Job drawing, mm, ordinate dimensions from the low corner. One solid piece. Round coordinates to 2 decimals unless told otherwise and drop trailing zeros. Order: outer loops, then holes, each group sorted by start corner. A loop starts at its lowest first (then second) coordinate and runs counter-clockwise, first axis right, second up. Notation, with made-up numbers: (-33.75, 82) -> (10.25, 82) arc R13 ccw to (10.25, 91) -> close; hole circle Ø6 at (14, 86). An arc over 180 degrees is marked (long way). Write item = value, one per line.
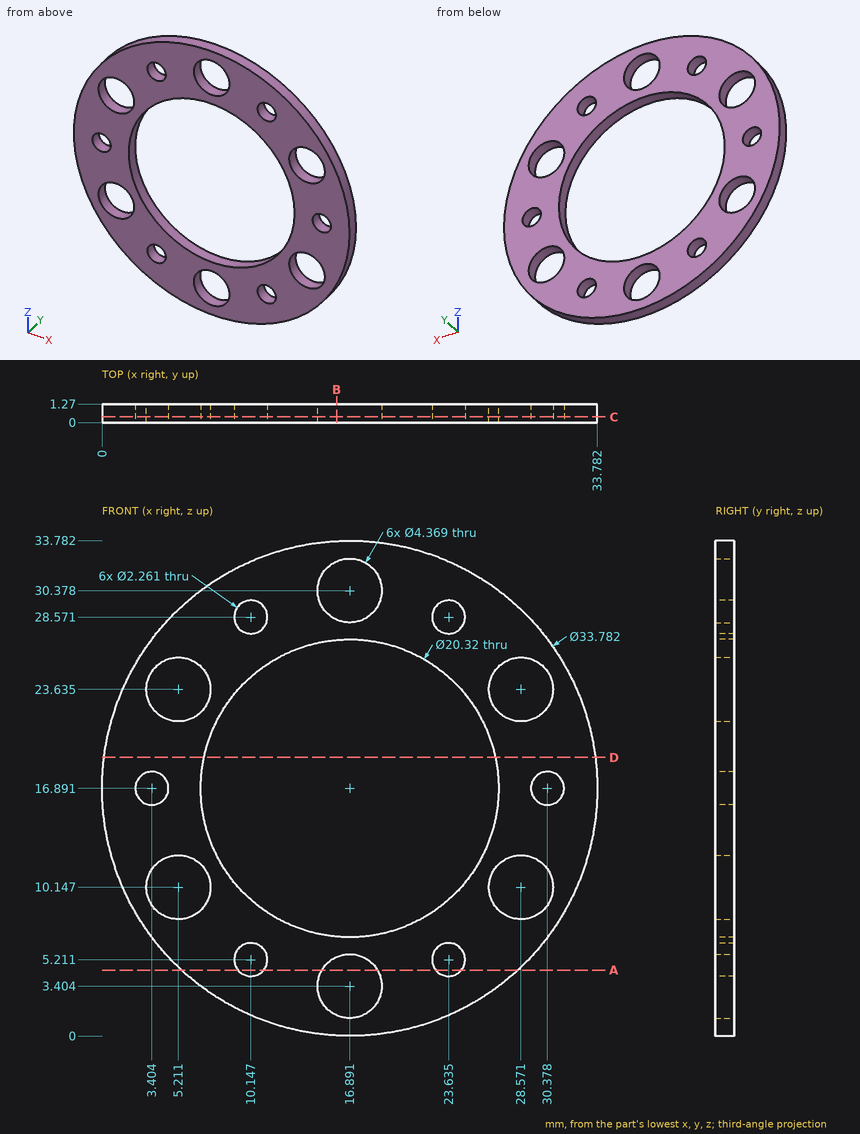
Q1. Cut at D-D, the plane z = 19. List the corners of the cut face in (x, y).
Check values:
outline = (0.13, 0) -> (6.95, 0) -> (6.95, 1.27) -> (0.13, 1.27) -> close; (26.83, 0) -> (33.65, 0) -> (33.65, 1.27) -> (26.83, 1.27) -> close
Q2. Cut at B-B, the plane x = 16. List the corners of the cut face in (y, z).
Check values:
outline = (0, 0.02) -> (1.27, 0.02) -> (1.27, 1.41) -> (0, 1.41) -> close; (0, 5.4) -> (1.27, 5.4) -> (1.27, 6.77) -> (0, 6.77) -> close; (0, 27.01) -> (1.27, 27.01) -> (1.27, 28.38) -> (0, 28.38) -> close; (0, 32.37) -> (1.27, 32.37) -> (1.27, 33.76) -> (0, 33.76) -> close
Q3. Probe probe 1 along X at (y, z) = (0.45, 10.5) (1 decimal); probe 2 along Z at (x, y) = (5, 1.2) (1 decimal); probe 3 along X at (y, z) = (0.9, 6) (1 decimal). List the from-to ranges inside material, lowest first.
Check values:
probe_1 = 1.3 to 3.1, 7.4 to 9, 24.8 to 26.4, 30.7 to 32.5
probe_2 = 4.9 to 8, 12.3 to 21.5, 25.8 to 28.9
probe_3 = 4 to 9.3, 11 to 22.8, 24.4 to 29.8
Q4. Flat gauge pin, fed straight in: pin 1 (2.5 mm diameter, centred on x = 30.38, z = 16.89, fed in from -Y). Where does the tip first touch, or does it go through?
Check values:
pin_1 = 0
Q5. Cut at C-C, the plane y = 0.4. Give the number of separate pieces and of enclosed holes in the cut face, and give its area (3 significant figures).
Check values:
separate_pieces = 1
enclosed_holes = 13
area = 458 mm²
Q6. Cut at A-A, the plane z = 4.5. List the corners of the cut face in (x, y) (1 decimal), and give its area (3 significant figures).
Check values:
outline = (5.4, 0) -> (9.3, 0) -> (9.3, 1.3) -> (5.4, 1.3) -> close; (11, 0) -> (15, 0) -> (15, 1.3) -> (11, 1.3) -> close; (18.8, 0) -> (22.8, 0) -> (22.8, 1.3) -> (18.8, 1.3) -> close; (24.5, 0) -> (28.4, 0) -> (28.4, 1.3) -> (24.5, 1.3) -> close
area = 19.9 mm²
